Build history of the part. All positions in model axes, mm. A direction names the side the tool comes from. Round coordinates to 2 decimals unless told otherwise and drop trailing zeros. Write each loop counter-clockwise with the first axis right and the second up, starting at its lowest first coordinate (ties: lowest second). Pieces come first, ordered by that corner, then holes. Notation, with made-up numbers: (16, -32.5) - (39, -32.5) arc R31 cw to (39, 3.5) - close; hole circle Ø5 at (37.25, 23.5). An arc over 180 degrees is marked (long way). Answer as a JSON object with one key per item and string values. Group by question number.
Item 1: Slice it at B-B, the plane x = 0. List the corners of the cut face in (y, z) (1 decimal), then the cut area to 3 significant figures.
Item 2: Probe line 1 (X direction, y = 8, z = 3.75) (3 decimals); line 2 (X direction, y = -11.5, z = 3) (3 decimals); line 3 (Z direction, x = -1, y = 11) (3 decimals). List the from-to ranges inside material, lowest first. Write a range as from..to.
Item 3: Flat gauge pins, fed straight in: pin 1 (1.6 mm diameter, centred on x = -21, z = 1, fed in from -Y); pin 2 (5 mm diameter, centred on x = -6, z = 8, fed in from -Y); pin 3 (3 mm diameter, centred on x = -0.5, y = -4, fed in from -Z); pin 4 (1.4 mm diameter, centred on y = -9, z = 4.76, fed in from -X). Where does each tip first touch, or does it go through?
Item 4: Two-plate mould, pull along X, no slides. Class faces 1 (the flat face through (22.225, 9, 3)), 2 (the flat face through (-19.05, 8, 3)), 3 (the flat face through (-22.225, 9, 3)), 4 (the cylindrical face through (0.04, -9.87, 4.96)): +X half, -X half, draft (parallel to the pull), parting line (faces both ways), or undercut.
Item 5: Which spindle directions (+Z, -Z, +X, -X, +Y, -Y) get a long thin tool onto all of the face, cutting with end or side? Do faces 5 (the flat face through (21, 0.952, 3)), 6 (the flat face through (0, 0, 0)), 7 (the flat face through (3.175, 0, 5)). Say none if no direction does.
Item 6: Slice it at D-D, the plane z = 4.5. Give the number of separate pieces and of enclosed holes in the cut face, then the cut area to 3 significant figures.
Item 7: Slice it at A-A, the plane y = 11. List the corners of the cut face in (x, z) (3 decimals), then the cut area to 3 significant figures.
from build123d import *

# Parameters (mm, degrees)
SKETCH1_W           = 6.35
SKETCH1_H           = 28.575
BOSS_EXTRUDE1_DEPTH = 9.525
SKETCH3_W           = 3.175
SKETCH3_H           = 13.335
BOSS_EXTRUDE2_DEPTH = 12.7
CUT_EXTRUDE1_REACH  = 34.262
SKETCH4_R           = 0.889


with BuildPart() as part:
    # Sketch1 → Boss-Extrude1 (new body)
    with BuildSketch(Plane.XY):
        Rectangle(SKETCH1_W, SKETCH1_H)
    extrude(amount=BOSS_EXTRUDE1_DEPTH)

    # Sketch3 → Boss-Extrude2 (add)
    with BuildSketch(Plane.XY.offset(9.525)):
        with Locations((-20.6375, 7.62)):
            Rectangle(SKETCH3_W, SKETCH3_H)
        Polygon((22.225, 17.4625), (-22.225, 17.4625), (-22.225, 14.2875), (-19.05, 14.2875), (-3.175, 14.2875), (3.175, 14.2875), (19.05, 14.2875), (22.225, 14.2875), align=None)
        with Locations((20.6375, 7.62)):
            Rectangle(SKETCH3_W, SKETCH3_H)
    extrude(amount=-BOSS_EXTRUDE2_DEPTH)

    # Sketch4 → Cut-Extrude1 (cut, up to next)
    with BuildSketch(Plane(origin=(3.175, 0, 0), x_dir=(0, 0, -1), z_dir=(1, 0, 0)), mode=Mode.PRIVATE) as cut_extrude1_sk1:
        with Locations((-4.7625, -9.0043)):
            Circle(SKETCH4_R)
    cut_extrude1_tool1 = extrude(cut_extrude1_sk1.sketch, amount=-CUT_EXTRUDE1_REACH, mode=Mode.PRIVATE) & part.part
    # Sketch4 → Cut-Extrude1 (cut, up to next)
    with BuildSketch(Plane(origin=(3.175, 0, 0), x_dir=(0, 0, -1), z_dir=(1, 0, 0)), mode=Mode.PRIVATE) as cut_extrude1_sk2:
        with Locations((-4.7625, 9.0043)):
            Circle(SKETCH4_R)
    cut_extrude1_tool2 = extrude(cut_extrude1_sk2.sketch, amount=-CUT_EXTRUDE1_REACH, mode=Mode.PRIVATE) & part.part
    add(cut_extrude1_tool1.solids().sort_by_distance((3.175, -9.0043, 4.7625))[0], mode=Mode.SUBTRACT)
    add(cut_extrude1_tool2.solids().sort_by_distance((3.175, 9.0043, 4.7625))[0], mode=Mode.SUBTRACT)


solid = part.part
Geometry says:
{
 "1": {"outline": "(-14.3, 0) - (14.3, 0) - (14.3, -3.2) - (17.5, -3.2) - (17.5, 9.5) - (-14.3, 9.5) - close; hole circle Ø1.8 at (-9, 4.8); hole circle Ø1.8 at (9, 4.8)", "area": "308 mm^2"},
 "2": {"line 1": "x = -22.225..-19.05, -3.175..3.175, 19.05..22.225", "line 2": "x = -3.175..3.175", "line 3": "z = 0..9.525"},
 "3": {"pin 1": "stops at y = 0.95", "pin 2": "stops at y = 14.29", "pin 3": "stops at z = 0", "pin 4": "passes through"},
 "4": {"face 1": "+X half", "face 2": "undercut", "face 3": "-X half", "face 4": "draft"},
 "5": {"face 5": "+Z, -Z, +X, -Y", "face 6": "-Z, -Y", "face 7": "+Z, -Z, -Y"},
 "6": {"separate pieces": "3", "enclosed holes": "0", "area": "386 mm^2"},
 "7": {"outline": "(-22.225, -3.175) - (-19.05, -3.175) - (-19.05, 9.525) - (-22.225, 9.525) - close; (-3.175, 0) - (3.175, 0) - (3.175, 9.525) - (-3.175, 9.525) - close; (19.05, -3.175) - (22.225, -3.175) - (22.225, 9.525) - (19.05, 9.525) - close", "area": "141 mm^2"}
}
